Check sheet for the modelled part. Datum: model origin and axes. Units: mm. A direction names the side the tool comes from. Round coordinates to 2 decimals unless told otherwise and drop trailing zeros. Loops run counter-clockwise (first coordinate to the right, second up) from the corner with the lowest first, then second, coordinate; pieces in that order, holes last. Notation, with made-up numbers: (-25, 70.25) -> (0, 70.25) arc R20 cw to (0, 97.25) -> close; hole circle Ø11 at (29, 3). An arc over 180 degrees is marked (long way). Return JSON: item names as keys, results as strings.
from build123d import *

# Parameters (mm, degrees)
SKETCH_1_W                = 211.717851242
SKETCH_1_H                = 121.662509304
EXTRUDE_1_DEPTH           = 10
SKETCH_2_W                = 5
SKETCH_2_H                = 15
EXTRUDE_2_DEPTH           = 40
CUT_EXTRUDE_1_DEPTH       = 129.477833404
CUT_EXTRUDE_1_DEPTH_BACK  = 129.477833404
SKETCH_3_OUTSIDE_W        = 263.568
SKETCH_3_OUTSIDE_H        = 173.512
SKETCH_4_W                = 15
SKETCH_4_H                = 15
EXTRUDE_3_DEPTH           = 10
CUT_EXTRUDE_2_DEPTH       = 130.428976448
CUT_EXTRUDE_2_DEPTH_BACK  = 5
SKETCH_5_W                = 251.048169007
SKETCH_5_H                = 208.83861988
CUT_EXTRUDE_3_DEPTH       = 97.900711095
CUT_EXTRUDE_3_DEPTH_BACK  = 97.900711095
SKETCH_7_R                = 4
SKETCH_8_W                = 6
SKETCH_8_H                = 22
EXTRUDE_6_DEPTH           = 6
CUT_EXTRUDE_4_DEPTH       = 128.58079771
CUT_EXTRUDE_4_DEPTH_BACK  = 128.58079771
SKETCH_10_W               = 17
SKETCH_10_H               = 6
EXTRUDE_7_DEPTH           = 5
SKETCH_11_R               = 11
EXTRUDE_8_DEPTH           = 0.6
SKETCH_12_R               = 6
EXTRUDE_9_DEPTH           = 7.4
CUT_EXTRUDE_10_DEPTH      = 116.586797735
CUT_EXTRUDE_10_DEPTH_BACK = 3
SKETCH_13_R               = 3
EXTRUDE_10_DEPTH          = 45
SKETCH_15_R               = 9.319080667
CUT_EXTRUDE_11_DEPTH      = 38
SKETCH_16_R               = 6
EXTRUDE_11_DEPTH          = 7.4
SKETCH_17_R               = 3
CUT_EXTRUDE_12_DEPTH      = 5
SKETCH_18_W               = 30
SKETCH_18_H               = 15
EXTRUDE_12_DEPTH          = 14.850514471
EXTRUDE_13_DEPTH          = 14.850514471
SKETCH_22_W               = 24
SKETCH_22_H               = 16.908951495
EXTRUDE_14_DEPTH          = 14.850514471
SKETCH_23_R               = 4.25
CUT_EXTRUDE_15_DEPTH      = 60
EXTRUDE_15_DEPTH          = 14.850514471
SKETCH_25_R               = 4.25
CUT_EXTRUDE_16_DEPTH      = 60
SKETCH_19_R               = 4.25
CUT_EXTRUDE_17_DEPTH      = 60
SKETCH_26_W               = 38.044769018
SKETCH_26_H               = 21.34609726
SKETCH_26_W_2             = 24.699869201
SKETCH_26_H_2             = 16.908951494
CUT_EXTRUDE_18_DEPTH      = 60
SKETCH_27_W               = 6.321147669
SKETCH_27_H               = 14.747228213
CUT_EXTRUDE_19_DEPTH      = 39


with BuildPart() as part:
    # 草图1 → 凸台-拉伸1 (new body)
    with BuildSketch(Plane(origin=(0, 0, 0), x_dir=(1, 0, 0), z_dir=(0, 1, 0))):
        Rectangle(SKETCH_1_W, SKETCH_1_H)
    extrude(amount=EXTRUDE_1_DEPTH)

    # 草图2 → 凸台-拉伸2 (add)
    with BuildSketch(Plane(origin=(0, 10, 0), x_dir=(1, 0, 0), z_dir=(0, 1, 0))):
        with Locations((-46.358925621, 47.311705854)):
            Rectangle(SKETCH_2_W, SKETCH_2_H)
        with Locations((-56.358925621, 47.311705854)):
            Rectangle(SKETCH_2_W, SKETCH_2_H)
        with Locations((-46.358925621, -47.688294146)):
            Rectangle(SKETCH_2_W, SKETCH_2_H)
        with Locations((-56.358925621, -47.688294146)):
            Rectangle(SKETCH_2_W, SKETCH_2_H)
    extrude(amount=EXTRUDE_2_DEPTH)

    # 草图3 outside → 切除-拉伸1 (cut, two sides: drawn at the far end of the back side and taken through both)
    with BuildSketch(Plane(origin=(0, 10, 0), x_dir=(1, 0, 0), z_dir=(0, 1, 0)).offset(-CUT_EXTRUDE_1_DEPTH_BACK)):
        Rectangle(SKETCH_3_OUTSIDE_W, SKETCH_3_OUTSIDE_H)
        Polygon((-105.858925621, 39.811705854), (-58.858925621, 39.811705854), (-58.858925621, 54.811705854), (-43.858925621, 54.811705854), (-43.858925621, 39.811705854), (-35.858925621, 39.811705854), (-35.858925621, -40.188294146), (-43.858925621, -40.188294146), (-43.858925621, -55.188294146), (-48.858925621, -55.188294146), (-48.858925621, -40.188294146), (-53.858925621, -40.188294146), (-53.858925621, -55.188294146), (-58.858925621, -55.188294146), (-58.858925621, -40.188294146), (-106.714815402, -40.188294146), align=None, mode=Mode.SUBTRACT)
    extrude(amount=CUT_EXTRUDE_1_DEPTH + CUT_EXTRUDE_1_DEPTH_BACK, mode=Mode.SUBTRACT)

    # 草图4 → 凸台-拉伸3 (add)
    with BuildSketch(Plane.XZ):
        with Locations((-51.358925621, 47.688294146)):
            Rectangle(SKETCH_4_W, SKETCH_4_H)
    extrude(amount=-EXTRUDE_3_DEPTH)

    # 草图5 → 切除-拉伸2 (cut, two sides: drawn at the far end of the back side and taken through both)
    with BuildSketch(Plane.XZ.offset(-CUT_EXTRUDE_2_DEPTH_BACK)):
        with Locations((-99.962010128, 39.987109066)):
            Rectangle(SKETCH_5_W, SKETCH_5_H)
    extrude(amount=CUT_EXTRUDE_2_DEPTH + CUT_EXTRUDE_2_DEPTH_BACK, mode=Mode.SUBTRACT)

    # 草图7 → 切除-拉伸3 (cut, two sides: drawn at the far end of the back side and taken through both)
    with BuildSketch(Plane(origin=(-43.858925621, 0, 0), x_dir=(0, 0, -1), z_dir=(1, 0, 0)).offset(-CUT_EXTRUDE_3_DEPTH_BACK)):
        with Locations((-50.188294146, 40)):
            Circle(SKETCH_7_R)
        with Locations((-50.188294146, 20)):
            Circle(SKETCH_7_R)
        with Locations((49.811705854, 40)):
            Circle(SKETCH_7_R)
        with Locations((49.811705854, 20)):
            Circle(SKETCH_7_R)
    extrude(amount=CUT_EXTRUDE_3_DEPTH + CUT_EXTRUDE_3_DEPTH_BACK, mode=Mode.SUBTRACT)

    # 草图8 → 凸台-拉伸6 (add)
    with BuildSketch(Plane.XZ.offset(-5)):
        with Locations((-32.858925621, 20.188294146)):
            Rectangle(SKETCH_8_W, SKETCH_8_H)
    extrude(amount=-EXTRUDE_6_DEPTH)

    # 草图9 → 切除-拉伸4 (cut, two sides: drawn at the far end of the back side and taken through both)
    with BuildSketch(Plane.XZ.offset(-5).offset(-CUT_EXTRUDE_4_DEPTH_BACK)):
        Polygon((-34.858925621, 39.188294146), (-34.858925621, 31.188294146), (-29.207793941, 25.537162465), (-29.207793941, 39.188294146), align=None)
    extrude(amount=CUT_EXTRUDE_4_DEPTH + CUT_EXTRUDE_4_DEPTH_BACK, mode=Mode.SUBTRACT)

    # 草图10 → 凸台-拉伸7 (add)
    with BuildSketch(Plane(origin=(-29.858925621, 0, 0), x_dir=(0, 0, -1), z_dir=(1, 0, 0))):
        Polygon((-31.188294146, 5), (-26.188294146, 5), (-26.188294146, 11), (-9.188294146, 11), (-9.188294146, 50), (-31.188294146, 50), align=None)
        with Locations((-17.688294146, 8)):
            Rectangle(SKETCH_10_W, SKETCH_10_H)
    extrude(amount=EXTRUDE_7_DEPTH)

    # 草图11 → 凸台-拉伸8 (add)
    with BuildSketch(Plane(origin=(-24.858925621, 0, 0), x_dir=(0, 0, -1), z_dir=(1, 0, 0))):
        with Locations((-20.188294146, 27.5)):
            Circle(SKETCH_11_R)
    extrude(amount=-EXTRUDE_8_DEPTH)

    # 草图12 → 凸台-拉伸9 (add)
    with BuildSketch(Plane(origin=(-24.858925621, 0, 0), x_dir=(0, 0, -1), z_dir=(1, 0, 0))):
        with Locations((-20.188294146, 27.5)):
            Circle(SKETCH_12_R)
    extrude(amount=EXTRUDE_9_DEPTH)

    # 草图13 → 切除-拉伸10 (cut, two sides: drawn at the far end of the back side and taken through both)
    with BuildSketch(Plane(origin=(-17.458925621, 0, 0), x_dir=(0, 0, -1), z_dir=(1, 0, 0)).offset(-CUT_EXTRUDE_10_DEPTH_BACK)):
        with Locations(Location((-20.188294146, 27.5, 0), (0, 0, 180))):
            Circle(SKETCH_13_R)
    extrude(amount=CUT_EXTRUDE_10_DEPTH + CUT_EXTRUDE_10_DEPTH_BACK, mode=Mode.SUBTRACT)

    # 草图14 → 凸台-拉伸10 (add)
    with BuildSketch(Plane(origin=(0, 5, 0), x_dir=(-1, 0, 0), z_dir=(0, -1, 0))):
        Polygon((34.858925621, -31.188294146), (29.858925621, -31.188294146), (29.858925621, -26.188294146), align=None)
    extrude(amount=-EXTRUDE_10_DEPTH)

    # 草图15 → 切除-拉伸11 (cut)
    with BuildSketch(Plane(origin=(-24.858925621, 0, 0), x_dir=(0, 0, -1), z_dir=(1, 0, 0))):
        with Locations((-20.188294146, 27.5)):
            Circle(SKETCH_15_R)
    extrude(amount=CUT_EXTRUDE_11_DEPTH, mode=Mode.SUBTRACT)

    # 草图16 → 凸台-拉伸11 (add)
    with BuildSketch(Plane(origin=(-24.858925621, 0, 0), x_dir=(0, 0, -1), z_dir=(1, 0, 0))):
        with Locations((-20.188294146, 30)):
            Circle(SKETCH_16_R)
    extrude(amount=EXTRUDE_11_DEPTH)

    # 草图17 → 切除-拉伸12 (cut)
    with BuildSketch(Plane(origin=(-17.458925621, 0, 0), x_dir=(0, 0, -1), z_dir=(1, 0, 0))):
        with Locations((-20.188294146, 30)):
            Circle(SKETCH_17_R)
    extrude(amount=-CUT_EXTRUDE_12_DEPTH, mode=Mode.SUBTRACT)

    # 草图18 → 凸台-拉伸12 (add)
    with BuildSketch(Plane(origin=(0, 10, 0), x_dir=(1, 0, 0), z_dir=(0, 1, 0))):
        with Locations((-90.858925621, 47.311705854)):
            Rectangle(SKETCH_18_W, SKETCH_18_H)
    extrude_12 = extrude(amount=-EXTRUDE_12_DEPTH)

    # 草图22 → 凸台-拉伸14 (add)
    with BuildSketch(Plane(origin=(0, 10, 0), x_dir=(1, 0, 0), z_dir=(0, 1, 0))):
        with Locations((-31.858925621, 48.266181602)):
            Rectangle(SKETCH_22_W, SKETCH_22_H)
    extrude_14 = extrude(amount=-EXTRUDE_14_DEPTH)

    # 草图23 → 切除-拉伸15 (cut)
    with BuildSketch(Plane(origin=(0, 10, 0), x_dir=(1, 0, 0), z_dir=(0, 1, 0))):
        with Locations(Location((-29.74274895, 45.141181602, 0), (0, 0, 270))):
            Circle(SKETCH_23_R)
    cut_extrude_15 = extrude(amount=-CUT_EXTRUDE_15_DEPTH, mode=Mode.SUBTRACT)

    # 草图24 → 凸台-拉伸15 (add)
    with BuildSketch(Plane(origin=(0, -4.850514471, 0), x_dir=(1, 0, 0), z_dir=(0, 1, 0))):
        Polygon((-43.858925621, -40.188294146), (-43.858925621, -57.09724564), (-19.74274895, -40.233286806), (-19.74274895, -40.188294146), align=None)
    extrude(amount=EXTRUDE_15_DEPTH)

    # 草图25 → 切除-拉伸16 (cut)
    with BuildSketch(Plane(origin=(0, 10, 0), x_dir=(1, 0, 0), z_dir=(0, 1, 0))):
        with Locations((-29.74274895, -45.517769893)):
            Circle(SKETCH_25_R)
    extrude(amount=-CUT_EXTRUDE_16_DEPTH, mode=Mode.SUBTRACT)

    # 草图19 → 切除-拉伸17 (cut)
    with BuildSketch(Plane(origin=(0, 10, 0), x_dir=(1, 0, 0), z_dir=(0, 1, 0))):
        with Locations(Location((-89.74274895, 45.141181602, 0), (0, 0, 270))):
            Circle(SKETCH_19_R)
    cut_extrude_17 = extrude(amount=-CUT_EXTRUDE_17_DEPTH, mode=Mode.SUBTRACT)


with BuildPart() as body_2:
    # 草图20 → 凸台-拉伸13 (new body)
    with BuildSketch(Plane(origin=(0, 10, 0), x_dir=(1, 0, 0), z_dir=(0, 1, 0))):
        Polygon((-105.858925621, -40.188294146), (-74.74274895, -56.834668943), (-74.74274895, -57.09724564), (-105.858925621, -57.09724564), align=None)
    extrude(amount=-EXTRUDE_13_DEPTH)


with BuildPart() as cut_extrude_18_tool:
    # 草图26 → 切除-拉伸18 (new body)
    with BuildSketch(Plane(origin=(0, 10, 0), x_dir=(1, 0, 0), z_dir=(0, 1, 0))):
        with Locations((-86.836541112, -50.861342776)):
            Rectangle(SKETCH_26_W, SKETCH_26_H)
        with Locations((-31.508991021, -48.642769893)):
            Rectangle(SKETCH_26_W_2, SKETCH_26_H_2)
    extrude(amount=-CUT_EXTRUDE_18_DEPTH)


with BuildPart() as part_1:
    add(part.part)

    # 切除-拉伸18: cut by cut_extrude_18_tool
    add(cut_extrude_18_tool.part, mode=Mode.SUBTRACT)

    # 镜向1: 凸台-拉伸12, 凸台-拉伸14, 切除-拉伸15, 切除-拉伸17 across plane
    add(extrude_12.mirror(Plane.XY))
    add(extrude_14.mirror(Plane.XY))
    add(cut_extrude_15.mirror(Plane.XY), mode=Mode.SUBTRACT)
    add(cut_extrude_17.mirror(Plane.XY), mode=Mode.SUBTRACT)

    # 草图27 → 切除-拉伸19 (cut)
    with BuildSketch(Plane(origin=(0, 50, 0), x_dir=(1, 0, 0), z_dir=(0, 1, 0))):
        with Locations((-33.019499456, -25.654978199)):
            Rectangle(SKETCH_27_W, SKETCH_27_H)
    extrude(amount=-CUT_EXTRUDE_19_DEPTH, mode=Mode.SUBTRACT)


with BuildPart() as body_2_1:
    add(body_2.part)

    # 切除-拉伸18: cut by cut_extrude_18_tool
    add(cut_extrude_18_tool.part, mode=Mode.SUBTRACT)


solid = part_1.part
Q1. Section check D-D (x = -64.5). Record the boundary of the cut face in (y, z), then the cut area to 3 significant figures.
Results list:
{"outline": "(5, -39.81) -> (10, -39.81) -> (10, 40.19) -> (5, 40.19) -> close", "area": "400 mm^2"}
Q2. Section check C-C (z = -15.5). Record the boundary of the cut face in (x, y).
Results list:
{"outline": "(-105.86, 5) -> (-35.86, 5) -> (-35.86, 10) -> (-105.86, 10) -> close"}
Q3. Material ranges on line 1 (Z direction, x = -55.8, y = 40); line 2 (X direction, y = 27, z = -41); line 3 (X direction, y = -0.5, z = -44), recorded low to high.
Results list:
{"line 1": "-54.81 to -53.81, -45.81 to -39.81, 40.19 to 46.19, 54.19 to 55.19", "line 2": "-58.86 to -53.86, -48.86 to -43.86", "line 3": "-105.86 to -93.84, -85.65 to -75.86, -43.86 to -33.84, -25.65 to -19.86"}
Q4. Go/stop test with flat-tipped pins: pin 1 (4 mm diameter, centred on x = -76, z = 28, fed in from -Y); pin 2 (4 mm diameter, centred on x = -68.5, y = 7, fed in from -Z); pin 3 (5.5 mm diameter, centred on x = -45.5, y = 37.5, fed in from -Z). Record where each tip stops, or that it passes through.
Results list:
{"pin 1": "y = 5", "pin 2": "z = -39.81", "pin 3": "z = -54.81"}
Q5. Section check A-A (y = 30). Record the boundary of the cut face in (x, z).
Results list:
{"outline": "(-58.86, -54.81) -> (-53.86, -54.81) -> (-53.86, -39.81) -> (-58.86, -39.81) -> close; (-58.86, 40.19) -> (-53.86, 40.19) -> (-53.86, 55.19) -> (-58.86, 55.19) -> close; (-48.86, -54.81) -> (-43.86, -54.81) -> (-43.86, -39.81) -> (-48.86, -39.81) -> close; (-48.86, 40.19) -> (-43.86, 40.19) -> (-43.86, 55.19) -> (-48.86, 55.19) -> close; (-29.86, 9.19) -> (-24.86, 9.19) -> (-24.86, 14.19) -> (-17.46, 14.19) -> (-17.46, 17.19) -> (-22.46, 17.19) -> (-22.46, 23.19) -> (-17.46, 23.19) -> (-17.46, 26.19) -> (-24.86, 26.19) -> (-24.86, 31.19) -> (-29.86, 31.19) -> close"}
Q6. Draft check along X on faces 5 (the flat face through (-56, 30, 40.188)), 6 (the cylindrical face through (-85.53, 2.68, 45.69)), 7 (the flat face through (-105.859, 6, 1)). Enter one of: released by +X, released by -X, zero draft, split by the parting line, or undercut.
Results list:
{"face 5": "zero draft", "face 6": "undercut", "face 7": "released by -X"}
Q7. Section check B-B (y = 8). Record the boundary of the cut face in (x, z).
Results list:
{"outline": "(-105.86, -54.81) -> (-75.86, -54.81) -> (-75.86, -39.81) -> (-58.86, -39.81) -> (-58.86, -54.81) -> (-43.86, -54.81) -> (-43.86, -56.72) -> (-19.86, -56.72) -> (-19.86, -39.81) -> (-35.86, -39.81) -> (-35.86, 9.19) -> (-24.86, 9.19) -> (-24.86, 31.19) -> (-35.86, 31.19) -> (-35.86, 39.81) -> (-19.86, 39.81) -> (-19.86, 56.72) -> (-43.86, 56.72) -> (-43.86, 55.19) -> (-58.86, 55.19) -> (-58.86, 40.19) -> (-75.86, 40.19) -> (-75.86, 54.81) -> (-105.86, 54.81) -> close; hole circle Ø8.5 at (-89.74, -45.14); hole circle Ø8.5 at (-89.74, 45.14); hole circle Ø8.5 at (-29.74, -45.14); hole circle Ø8.5 at (-29.74, 45.14)"}
Q8. Tool access check on faces 1 (the flat face through (-53.859, 30, -47)), 2 (the flat face through (-24.859, 23, 20)), 3 (the flat face through (-28, 27, 31.188)), 4 (the flat face through (-43.859, 30, -47)). Record the directions out of +Z, -Z, +X, -X, +Y, -Y that give a thin tool (end or side, any length) a straight path to the whole face; none if there is none.
Results list:
{"face 1": "+Z, -Z, +Y", "face 2": "+X", "face 3": "+X, +Y, -Y", "face 4": "+Z, -Z, +X, +Y"}
